Design review of the part built by this model. Coordinates are the model's own, in mm. Face numbers are marked on the shaded views. A direction names the side the tool comes from. Coordinates: 2 decimals unless noted, no trailing zeros. Loops run counter-clockwise (first coordinate to the right, second up) from the corner with the lowest first, then second, coordinate; pieces in that order, holes last.
Q1. Add section A-A on y = -11. Give the boundary of the cut face in (x, z), and give its area (3 significant figures).
Q2. Machinability: for the marked faces 1, 2 and 3, which of the approach directions +Z, -Z, +X, -X, +Y, -Y give a long, thin tool a straight path to every point of the face, cutting with its end or side? Answer none if there is none.
Q3. Add section B-B on x = 6. Give the boundary of the cut face in (y, z), and give its area (3 significant figures).
Q4. Add section C-C on z = 13. Give the boundary of the cut face in (x, y).
Q5. For P1, Ø4, axis at y = -10, z = 14, coming from the +X side; P2, Ø1, axis at x = 4.5, z = 8.5, coming from the +Y side; P3, Ø2.5, axis at y = -13.5, z = 8, coming from the -X side; P4, Ø3, axis at y = -10, z = 10, coming from the +X side, all flat-tipped, find the tip position at first contact; note any pin that passes through.
Q6. Wall thickness on probe 1 along X at (y, z) = (-22, 13.75); probe 2 along Z at (x, y) = (5.75, -5.5); probe 3 along Z at (x, y) = (1.25, -18): over which ranges is each line inside the solid? List them lowest first.
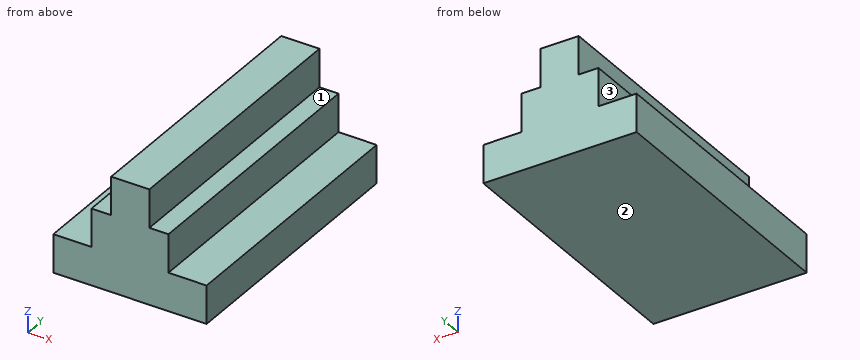
```python
from build123d import *

# Parameters (mm, degrees)
F0_W     = 2.5
F0_H     = 5
F1_DEPTH = 35


with BuildPart() as f1:
    # F0 (on Front) → F1 (new body)
    with BuildSketch(Plane.XZ):
        with Locations((-3.75, 13.401443)):
            Rectangle(F0_W, F0_H)
        with Locations((-1.25, 13.401443)):
            Rectangle(F0_W, F0_H)
        Polygon((-2.5, 10.901443), (-5, 10.901443), (-7.576827, 10.901443), (-7.576827, 5.901443), (-12.576827, 5.901443), (-12.576827, 0.901443), (7.5, 0.901443), (7.5, 5.901443), (2.5, 5.901443), (2.5, 10.901443), (0, 10.901443), align=None)
    extrude(amount=F1_DEPTH)


solid = f1.part
```
Entries:
1. outline: (-12.58, 0.9) - (7.5, 0.9) - (7.5, 5.9) - (2.5, 5.9) - (2.5, 10.9) - (0, 10.9) - (0, 15.9) - (-5, 15.9) - (-5, 10.9) - (-7.58, 10.9) - (-7.58, 5.9) - (-12.58, 5.9) - close
1. area: 176 mm2
2. face 1: +Z, +X, +Y, -Y
2. face 2: -Z, +X, -X, +Y, -Y
2. face 3: +Z, -X, +Y, -Y
3. outline: (-35, 0.9) - (0, 0.9) - (0, 5.9) - (-35, 5.9) - close
3. area: 175 mm2
4. outline: (-5, -35) - (0, -35) - (0, 0) - (-5, 0) - close
5. P1: stops at x = 0
5. P2: passes through
5. P3: stops at x = -7.58
5. P4: stops at x = 2.5
6. probe 1: x = -5 to 0
6. probe 2: z = 0.9 to 5.9
6. probe 3: z = 0.9 to 10.9
